from build123d import *

# Parameters (mm, degrees)
SKETCH3_W           = 30
SKETCH3_H           = 72.5
BOSS_EXTRUDE2_DEPTH = 15.95
SKETCH7_W           = 20.5
SKETCH7_H           = 41
CUT_EXTRUDE5_DEPTH  = 8.1
SKETCH8_W           = 30
SKETCH8_H           = 35
CUT_EXTRUDE6_DEPTH  = 9.95
CUT_EXTRUDE7_DEPTH  = 50.683649222
SKETCH10_R          = 3.1
CUT_EXTRUDE8_DEPTH  = 50.683649222
CUT_EXTRUDE9_REACH  = 44.349
SKETCH11_R          = 1.6
CUT_EXTRUDE10_REACH = 42.996
SKETCH12_R          = 1.6
SKETCH13_W          = 7
SKETCH13_H          = 7
SKETCH13_R          = 1.6
BOSS_EXTRUDE3_DEPTH = 4
CUT_EXTRUDE11_DEPTH = 0.5


with BuildPart() as part:
    # Sketch3 → Boss-Extrude2 (new body)
    with BuildSketch(Plane(origin=(0, 0, 0), x_dir=(1, 0, 0), z_dir=(0, 1, 0))):
        Rectangle(SKETCH3_W, SKETCH3_H)
    extrude(amount=BOSS_EXTRUDE2_DEPTH)

    # Sketch7 → Cut-Extrude5 (cut)
    with BuildSketch(Plane.XZ):
        with Locations((0, 9)):
            Rectangle(SKETCH7_W, SKETCH7_H)
    extrude(amount=-CUT_EXTRUDE5_DEPTH, mode=Mode.SUBTRACT)

    # Sketch8 → Cut-Extrude6 (cut)
    with BuildSketch(Plane(origin=(0, 15.95, 0), x_dir=(1, 0, 0), z_dir=(0, 1, 0))):
        with Locations((0, 1.25)):
            Rectangle(SKETCH8_W, SKETCH8_H)
    extrude(amount=-CUT_EXTRUDE6_DEPTH, mode=Mode.SUBTRACT)

    # Sketch9 → Cut-Extrude7 (cut, through all)
    with BuildSketch(Plane(origin=(15, 0, 0), x_dir=(0, 0, -1), z_dir=(1, 0, 0))):
        Polygon((-36.25, 15.95), (-33.75, 15.95), (-33.75, 9.05), (-27.25, 9.05), (-27.25, 4.05), (-36.25, 4.05), align=None)
    extrude(amount=-CUT_EXTRUDE7_DEPTH, mode=Mode.SUBTRACT)

    # Sketch10 → Cut-Extrude8 (cut, through all)
    with BuildSketch(Plane(origin=(15, 0, 0), x_dir=(0, 0, -1), z_dir=(1, 0, 0))):
        with Locations((24.25, 16)):
            Circle(SKETCH10_R)
        with Locations((-21.75, 16)):
            Circle(SKETCH10_R)
    extrude(amount=-CUT_EXTRUDE8_DEPTH, mode=Mode.SUBTRACT)

    # Sketch11 → Cut-Extrude9 (cut, up to next)
    with BuildSketch(Plane(origin=(0, 15.95, 0), x_dir=(1, 0, 0), z_dir=(0, 1, 0)), mode=Mode.PRIVATE) as cut_extrude9_sk1:
        with Locations(Location((-9.5, -30.25, 0), (0, 0, 270))):
            Circle(SKETCH11_R)
    cut_extrude9_tool1 = extrude(cut_extrude9_sk1.sketch, amount=-CUT_EXTRUDE9_REACH, mode=Mode.PRIVATE) & part.part
    # Sketch11 → Cut-Extrude9 (cut, up to next)
    with BuildSketch(Plane(origin=(0, 15.95, 0), x_dir=(1, 0, 0), z_dir=(0, 1, 0)), mode=Mode.PRIVATE) as cut_extrude9_sk2:
        with Locations(Location((9.5, -30.25, 0), (0, 0, 270))):
            Circle(SKETCH11_R)
    cut_extrude9_tool2 = extrude(cut_extrude9_sk2.sketch, amount=-CUT_EXTRUDE9_REACH, mode=Mode.PRIVATE) & part.part
    # Sketch11 → Cut-Extrude9 (cut, up to next)
    with BuildSketch(Plane(origin=(0, 15.95, 0), x_dir=(1, 0, 0), z_dir=(0, 1, 0)), mode=Mode.PRIVATE) as cut_extrude9_sk3:
        with Locations(Location((-9.5, 30, 0), (0, 0, 270))):
            Circle(SKETCH11_R)
    cut_extrude9_tool3 = extrude(cut_extrude9_sk3.sketch, amount=-CUT_EXTRUDE9_REACH, mode=Mode.PRIVATE) & part.part
    # Sketch11 → Cut-Extrude9 (cut, up to next)
    with BuildSketch(Plane(origin=(0, 15.95, 0), x_dir=(1, 0, 0), z_dir=(0, 1, 0)), mode=Mode.PRIVATE) as cut_extrude9_sk4:
        with Locations(Location((9.5, 30, 0), (0, 0, 270))):
            Circle(SKETCH11_R)
    cut_extrude9_tool4 = extrude(cut_extrude9_sk4.sketch, amount=-CUT_EXTRUDE9_REACH, mode=Mode.PRIVATE) & part.part
    add(cut_extrude9_tool1.solids().sort_by_distance((-9.5, 15.95, 30.25))[0], mode=Mode.SUBTRACT)
    add(cut_extrude9_tool2.solids().sort_by_distance((9.5, 15.95, 30.25))[0], mode=Mode.SUBTRACT)
    add(cut_extrude9_tool3.solids().sort_by_distance((-9.5, 15.95, -30))[0], mode=Mode.SUBTRACT)
    add(cut_extrude9_tool4.solids().sort_by_distance((9.5, 15.95, -30))[0], mode=Mode.SUBTRACT)

    # Sketch12 → Cut-Extrude10 (cut, up to next)
    with BuildSketch(Plane(origin=(0, 4.05, 0), x_dir=(1, 0, 0), z_dir=(0, 1, 0)), mode=Mode.PRIVATE) as cut_extrude10_sk1:
        with Locations(Location((-5, -33, 0), (0, 0, 270))):
            Circle(SKETCH12_R)
    cut_extrude10_tool1 = extrude(cut_extrude10_sk1.sketch, amount=-CUT_EXTRUDE10_REACH, mode=Mode.PRIVATE) & part.part
    # Sketch12 → Cut-Extrude10 (cut, up to next)
    with BuildSketch(Plane(origin=(0, 4.05, 0), x_dir=(1, 0, 0), z_dir=(0, 1, 0)), mode=Mode.PRIVATE) as cut_extrude10_sk2:
        with Locations(Location((5, -33, 0), (0, 0, 270))):
            Circle(SKETCH12_R)
    cut_extrude10_tool2 = extrude(cut_extrude10_sk2.sketch, amount=-CUT_EXTRUDE10_REACH, mode=Mode.PRIVATE) & part.part
    # Sketch12 → Cut-Extrude10 (cut, up to next)
    with BuildSketch(Plane(origin=(0, 4.05, 0), x_dir=(1, 0, 0), z_dir=(0, 1, 0)), mode=Mode.PRIVATE) as cut_extrude10_sk3:
        with Locations(Location((-5, 15, 0), (0, 0, 270))):
            Circle(SKETCH12_R)
    cut_extrude10_tool3 = extrude(cut_extrude10_sk3.sketch, amount=-CUT_EXTRUDE10_REACH, mode=Mode.PRIVATE) & part.part
    # Sketch12 → Cut-Extrude10 (cut, up to next)
    with BuildSketch(Plane(origin=(0, 4.05, 0), x_dir=(1, 0, 0), z_dir=(0, 1, 0)), mode=Mode.PRIVATE) as cut_extrude10_sk4:
        with Locations(Location((5, 15, 0), (0, 0, 270))):
            Circle(SKETCH12_R)
    cut_extrude10_tool4 = extrude(cut_extrude10_sk4.sketch, amount=-CUT_EXTRUDE10_REACH, mode=Mode.PRIVATE) & part.part
    add(cut_extrude10_tool1.solids().sort_by_distance((-5, 4.05, 33))[0], mode=Mode.SUBTRACT)
    add(cut_extrude10_tool2.solids().sort_by_distance((5, 4.05, 33))[0], mode=Mode.SUBTRACT)
    add(cut_extrude10_tool3.solids().sort_by_distance((-5, 4.05, -15))[0], mode=Mode.SUBTRACT)
    add(cut_extrude10_tool4.solids().sort_by_distance((5, 4.05, -15))[0], mode=Mode.SUBTRACT)

    # Sketch13 → Boss-Extrude3 (add)
    # profile 1 of 2: a face of its own
    with BuildSketch(Plane(origin=(0, 0, -36.25), x_dir=(-1, 0, 0), z_dir=(0, 0, -1))):
        with Locations((18.5, 12.45)):
            Rectangle(SKETCH13_W, SKETCH13_H)
        with Locations((18.5, 12.45)):
            Circle(SKETCH13_R, mode=Mode.SUBTRACT)
    # profile 2 of 2: a face of its own
    with BuildSketch(Plane(origin=(0, 0, -36.25), x_dir=(-1, 0, 0), z_dir=(0, 0, -1))):
        with Locations((-18.5, 12.45)):
            Rectangle(SKETCH13_W, SKETCH13_H)
        with Locations((-18.5, 12.45)):
            Circle(SKETCH13_R, mode=Mode.SUBTRACT)
    extrude(amount=-BOSS_EXTRUDE3_DEPTH)

    # Sketch14 → Cut-Extrude11 (cut, symmetric)
    with BuildSketch(Plane(origin=(0, 0, 0), x_dir=(0, 0, -1), z_dir=(1, 0, 0))):
        Polygon((18.3, 0), (11.5, 0), (11.5, 1.5), align=None)
        Polygon((-36.3, 0), (-29.5, 1.5), (-29.5, 0), align=None)
    extrude(amount=CUT_EXTRUDE11_DEPTH, both=True, mode=Mode.SUBTRACT)


solid = part.part
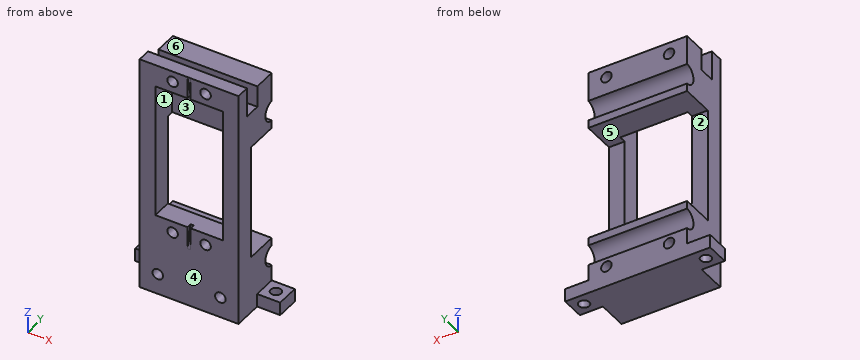
The model under review builds one solid part; all positions refer to its coordinate system, in mm. Face numbers are marked on the shaded views. A direction names the side the tool comes from. Round coordinates to 2 decimals unless told otherwise and drop trailing zeros. Order: outer loops, then holes, each group sorted by start corner. A loop starts at its lowest first (then second) coordinate and runs counter-clockwise, first axis right, second up. Notation, with made-up numbers: (30, -10.75) -> (50, -10.75) arc R16 ccw to (50, -6.75) -> close; hole circle Ø1 at (-38, 59.25). An arc over 180 degrees is marked (long way). Use CSV: the item, a comma, the result in double quotes. Start each with the question number.
(1) Consider section C-C on z = -1. Write out the cut boundary in (x, y).
(2) Insertion check: pin 1 (1.2 mm diameter, centred on x = 19.5, z = -33.5, fed in from -Y); pin 2 (1.5 mm diameter, centred on x = -0.5, z = 26, fed in from -Y); pin 3 (2 mm diameter, centred on x = -17.5, y = 13.5, fed in from +Z). Each pin has a flat end and moves straight along its axis. Give the tip position at first contact, or say it passes through.
(3) Mouldability with a two-part tool opening along X and no side actions: class the marked faces 1, 2 and 3 as pulls with the +X half, pulls with the -X half, needs draft (parallel to the pull), parting line crosses it, or undercut.
(4) Consider section B-B on y = 5. Write out the cut boundary in (x, z).
(5) Tool access review of the marked faces 4, 5 and 6: name each direction out of +Z, -Z, +X, -X, +Y, -Y from which nothing blocks a thin tool from reaching the whole face with its end or side.
(6) Consider section D-D on x = -18.5. Write out the cut boundary in (y, z).
(7) Wall thickness on probe 1 along X at (y, z) = (2.3, 33); probe 2 along Y at (x, z) = (-18.5, -33.25); probe 3 along X at (y, z) = (8, 17.5): over which ranges is each line inside the solid? List them lowest first. Write a range as from..to.
(8) Consider section A-A on x = -9.5. Write out the cut boundary in (y, z), and give its area (3 significant figures).
Responses:
1,outline,"(-15, 0) -> (-10.25, 0) -> (-10.25, 6) -> (-15, 6) -> close; (10.25, 0) -> (15, 0) -> (15, 6) -> (10.25, 6) -> close"
2,pin 1,"y = 8.95"
2,pin 2,"y = 8.1"
2,pin 3,"z = -32.25"
3,face 1,"undercut"
3,face 2,"needs draft"
3,face 3,"undercut"
4,outline,"(-15, -36.25) -> (15, -36.25) -> (15, 27.25) -> (10.25, 27.25) -> (10.25, -11.5) -> (-10.25, -11.5) -> (-10.25, 27.25) -> (-15, 27.25) -> close; hole circle Ø3.2 at (-9.5, -30); hole circle Ø3.2 at (9.5, -30)"
5,face 4,"+Z, -Z, +X, -X, -Y"
5,face 5,"+X, -X, +Y"
5,face 6,"+Z, +X, -X, +Y"
6,outline,"(8.95, -36.25) -> (10.85, -36.25) -> (10.85, -32.25) -> (8.95, -32.25) -> close; (14.05, -36.25) -> (15.95, -36.25) -> (15.95, -32.25) -> (14.05, -32.25) -> close"
7,probe 1,"-15..-6.6, -3.4..3.4, 6.6..15"
7,probe 2,"8.95..10.85, 14.05..15.95"
7,probe 3,"-15..-10.25, 10.25..15"
8,outline,"(0, -36.25) -> (15.95, -36.25) -> (15.95, -31.6) -> (0, -31.6) -> close; (0, -28.4) -> (15.95, -28.4) -> (15.95, -27.35) arc R3.1 cw to (15.95, -21.15) -> (15.95, -18.75) -> (6, -18.75) -> (6, -11.5) -> (0, -11.5) -> close; (0, 29.5) -> (4.05, 29.5) -> (4.05, 36.25) -> (0, 36.25) -> close; (8.1, 16.25) -> (15.95, 16.25) -> (15.95, 18.65) arc R3.1 cw to (15.95, 24.85) -> (15.95, 28.65) -> (9.05, 28.65) -> (9.05, 27.25) -> (8.1, 27.25) -> close; (9.05, 31.85) -> (15.95, 31.85) -> (15.95, 33.75) -> (9.05, 33.75) -> close"
8,area,"378 mm²"
